Work out the finished part from the listing and answer in its coordinate system (mm). Give positions to 0.01 mm unless a question says otherwise; leave off trailing zeros. Write each loop counter-clockwise with the first axis right and the second up, starting at its lowest first coordinate (ties: lowest second). Pieces come first, ordered by that corner, then holes. Notation, with made-up numbers: (64.5, 58) - (81.5, 58) arc R16 ccw to (81.5, 67) - close; hole circle Ø1 at (51.5, -25). An arc over 180 degrees is marked (long way). Write item = value, one per line.
Autodesk Inventor part; units mm, degrees
ref_plane "YZ Plane" through (0, 0, 0) normal (1, 0, 0) x (0, 1, 0)
ref_plane "XZ Plane" through (0, 0, 0) normal (0, 1, 0) x (-1, 0, 0)
ref_plane "XY Plane" through (0, 0, 0) normal (0, 0, 1) x (1, 0, 0)
sketch "Boceto1" plane through (0, 0, 0) normal (0, 1, 0) x (-1, 0, 0)
  arc A0 (30.25, 0) -> (-30.25, 0) centre (0, 0) ccw
  circle A1 centre (0, 0) radius 81.4 construction
  line L0 (66, 0) -> (30.25, 0)
  line L1 (-30.25, 0) -> (-66, 0)
  line L2 (0, 0) -> (103.5194, 0) construction
  line L3 (73.1993, 73.1993) -> (0, 0) construction
  line L4 (0, 0) -> (-73.1993, 73.1993) construction
  line L5 (0, 0) -> (103.5194, 0) construction
  line L6 (66, 66) -> (36.5996, 36.5996) construction
  line L7 (56.6662, 66) -> (41.7682, 51.102)
  line L8 (51.102, 41.7682) -> (66, 56.6662)
  arc A2 (66, 56.6662) -> (56.6662, 66) centre (61.3331, 61.3331) ccw
  line L9 (0, 0) -> (0, 91.3472) construction
  line L10 (-56.6662, 66) -> (-41.7682, 51.102)
  line L11 (-51.102, 41.7682) -> (-66, 56.6662)
  arc A3 (-56.6662, 66) -> (-66, 56.6662) centre (-61.3331, 61.3331) ccw
  circle A4 centre (61.3331, 61.3331) radius 2.75
  circle A5 centre (-61.3331, 61.3331) radius 2.75
  arc A6 (66, 0) -> (51.102, 41.7682) centre (0, 0) ccw
  arc A7 (41.7682, 51.102) -> (-41.7682, 51.102) centre (0, 0) ccw
  arc A8 (-51.102, 41.7682) -> (-66, 0) centre (0, 0) ccw
  point P0 (36.5996, 45.9334)
  point P1 (45.9334, 36.5996)
  point P2 (51.2998, 51.2998)
  point P3 (-36.5996, 45.9334)
  point P4 (-45.9334, 36.5996)
  dimension "d9" = 5.5
  dimension "d11" = 5.5
extrude "Extrusión2" add sketch "Boceto1" along normal blind 2
properties part number "Rail"
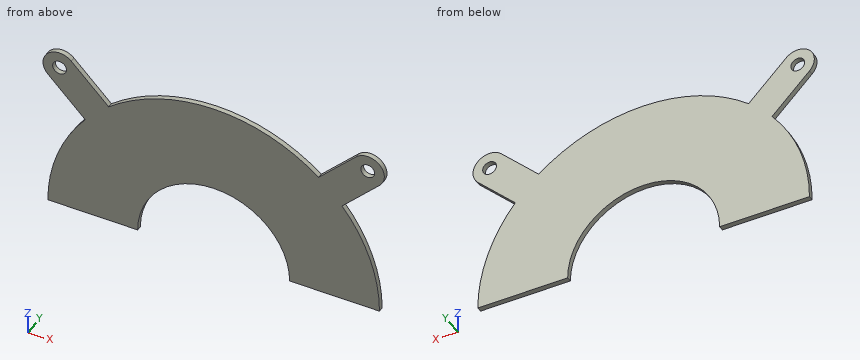
1. Find section C-C, the plane x = 0. Give the vertices of the cut face in (y, z).
Solution:
outline = (0, 30.25) - (2, 30.25) - (2, 66) - (0, 66) - close
2. Find section A-A, the plane z = 12. Give the vertices of the cut face in (x, y).
Solution:
outline = (-64.9, 0) - (-27.77, 0) - (-27.77, 2) - (-64.9, 2) - close; (27.77, 0) - (64.9, 0) - (64.9, 2) - (27.77, 2) - close
3. Given pin 1 (1 mm diameter, centred on x = 16.5, y = 1.5, fed in from +Z); pin 2 (4.5 mm diameter, centred on x = 61.33, z = 61.33, fed in from +Y), each flat-ended and moving along its own axis, determine where each tip first touches the part or whether it passes through.
Solution:
pin_1 = 64.03
pin_2 = through
4. Find section B-B, the plane y = 0.9. Give the vertices of the cut face in (x, z), then the cut area to 3 significant figures.
Solution:
outline = (-66, 0) - (-30.25, 0) arc R30.25 cw to (30.25, 0) - (66, 0) arc R66 ccw to (51.1, 41.77) - (66, 56.67) arc R6.6 ccw to (56.67, 66) - (41.77, 51.1) arc R66 ccw to (-41.77, 51.1) - (-56.67, 66) arc R6.6 ccw to (-66, 56.67) - (-51.1, 41.77) arc R66 ccw to start; hole circle Ø5.5 at (-61.33, 61.33); hole circle Ø5.5 at (61.33, 61.33)
area = 6,040 mm^2
5. Find section D-D, the plane x = -19.5. Give the vertices of the cut face in (y, z).
Solution:
outline = (0, 23.13) - (2, 23.13) - (2, 63.05) - (0, 63.05) - close
6. Straight lines are drawn through the part: line 1 (X direction, y = 0.65, z = 55.5); line 2 (X direction, y = 0.6, z = 53.5); line 3 (X direction, y = 0.65, z = 20.5). For each, find the intervals that lie inside material, in ascending order.
Solution:
line_1 = -64.83 to -46.17, -35.72 to 35.72, 46.17 to 64.83
line_2 = -62.83 to -44.17, -38.65 to 38.65, 44.17 to 62.83
line_3 = -62.74 to -22.24, 22.24 to 62.74
